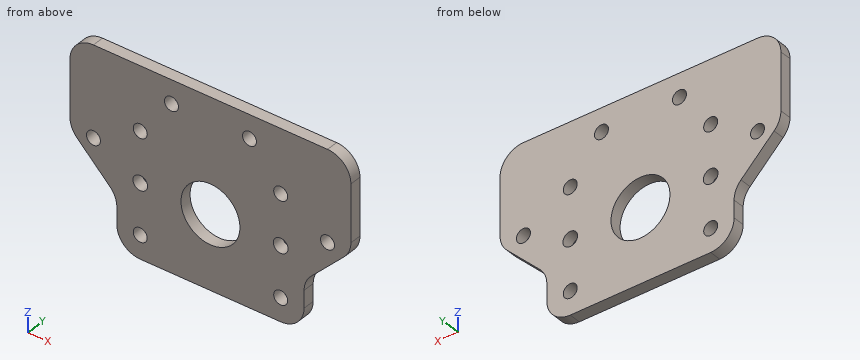
from build123d import *

# Parameters (mm, degrees)
SKETCH1_R           = 8
BOSS_EXTRUDE1_DEPTH = 3.175
SKETCH2_R           = 1.9939
CUT_EXTRUDE1_DEPTH  = 4.175
SKETCH14_R          = 1.89865
M3_TAP_DEPTH        = 4.175
SKETCH15_R          = 1.89865
M5_THROUGH_DEPTH    = 4.175
CUT_EXTRUDE2_DEPTH  = 4.175
FILLET2_R           = 6.35


with BuildPart() as part:
    # Sketch1 → Boss-Extrude1 (new body)
    with BuildSketch(Plane(origin=(0, 0, 0), x_dir=(1, 0, 0), z_dir=(0, 1, 0))):
        Polygon((0, 0), (76.2, 0), (76.2, 50.8), (38.1, 50.8), (0, 50.8), align=None)
        with Locations((38.1, 30.8)):
            Circle(SKETCH1_R, mode=Mode.SUBTRACT)
    extrude(amount=BOSS_EXTRUDE1_DEPTH)

    # Sketch2 → Cut-Extrude1 (cut, through all)
    with BuildSketch(Plane(origin=(0, 3.175, 0), x_dir=(1, 0, 0), z_dir=(0, 1, 0))):
        with Locations((19.05, 30.8)):
            Circle(SKETCH2_R)
        with Locations((57.15, 30.8)):
            Circle(SKETCH2_R)
    extrude(amount=-CUT_EXTRUDE1_DEPTH, mode=Mode.SUBTRACT)

    # Sketch14 → M3-tap (cut, through all)
    with BuildSketch(Plane.XZ):
        with Locations((57.15, -44.45)):
            Circle(SKETCH14_R)
        with Locations((19.05, -44.45)):
            Circle(SKETCH14_R)
        with Locations((19.05, -17.15)):
            Circle(SKETCH14_R)
        with Locations((57.15, -17.15)):
            Circle(SKETCH14_R)
    extrude(amount=-M3_TAP_DEPTH, mode=Mode.SUBTRACT)

    # Sketch15 → M5-through (cut, through all)
    with BuildSketch(Plane.XZ):
        with Locations((69.85, -24.45004)):
            Circle(SKETCH15_R)
        with Locations((48.683333333, -6.35)):
            Circle(SKETCH15_R)
        with Locations((27.516666667, -6.35)):
            Circle(SKETCH15_R)
        with Locations((6.35, -24.45004)):
            Circle(SKETCH15_R)
    extrude(amount=-M5_THROUGH_DEPTH, mode=Mode.SUBTRACT)

    # Sketch12 → Cut-Extrude2 (cut, through all)
    with BuildSketch(Plane(origin=(0, 3.175, 0), x_dir=(1, 0, 0), z_dir=(0, 1, 0))):
        Polygon((0, 50.8), (12.7, 50.8), (12.7, 37.15), (0, 24.45), align=None)
        Polygon((63.5, 50.8), (63.5, 37.15), (76.2, 24.45), (76.2, 50.8), align=None)
    extrude(amount=-CUT_EXTRUDE2_DEPTH, mode=Mode.SUBTRACT)

    # Fillet2
    fillet2_edges = [part.edges().sort_by_distance(p)[0] for p in [
        (0, 1.5875, -24.45),
        (12.7, 1.5875, -50.8),
        (12.7, 1.5875, -37.15),
        (63.5, 1.5875, -50.8),
        (76.2, 1.5875, -24.45),
        (63.5, 1.5875, -37.15),
        (76.2, 1.5875, 0),
        (0, 1.5875, 0),
    ]]
    fillet(fillet2_edges, radius=FILLET2_R)


solid = part.part
For this review, take the finished solid that the model builds, in its own axes (mm). Give positions to 0.01 mm unless a question says otherwise; leave off trailing zeros. Order: outer loops, then holes, each group sorted by start corner. A loop starts at its lowest first (then second) coordinate and runs counter-clockwise, first axis right, second up. Notation, with made-up numbers: M 62,36.5 L 82,36.5 A5 ccw 82,45.5 Z; hole C 48,-24 d9. An arc over 180 degrees is marked long. Answer in a Markdown table with one row per item. Add a question column.
(1) For pin 1 (1 mm diameter, centred on y = 1.5, z = -41, fed in from -X); pin 2 (1 mm diameter, centred on y = 2, z = -42, fed in from +X), all flat-tipped, find the tip position at first contact; note any pin that passes through.
(2) Consider section C-C on z = -17.15. State the section outline as (x, y) points (3 decimals).
(3) Wall thickness on probe 1 along Z at (x, y) = (19.05, 0.85); probe 2 along X at (y, z) = (1.45, -6.5); probe 3 along X at (y, z) = (1.15, -30): over which ranges is each line inside the solid? List them lowest first. Write a range as [from, to].
(4) Consider section A-A on z = -30.8. State the section outline as (x, y) points (3 decimals), and give its area (3 significant figures).
(5) Consider section B-B on x = 33. State the section outline as (y, z) points (3 decimals).
(6) Consider section D-D on y = 2.6. Give the number of separate pieces and of enclosed holes in the cut face, and give its area (3 significant figures).
Evaluation:
| question | item | result |
|---|---|---|
| 1 | pin 1 | stops at x = 12.7 |
| 1 | pin 2 | stops at x = 63.5 |
| 2 | outline | M 0,0 L 17.151,0 L 17.151,3.175 L 0,3.175 Z; M 20.949,0 L 55.251,0 L 55.251,3.175 L 20.949,3.175 Z; M 59.049,0 L 76.2,0 L 76.2,3.175 L 59.049,3.175 Z |
| 3 | probe 1 | z = [-50.8, -46.35], [-42.55, -32.79], [-28.81, -19.05], [-15.25, 0] |
| 3 | probe 2 | x = [0, 25.62], [29.41, 46.79], [50.58, 76.2] |
| 3 | probe 3 | x = [5.55, 17.22], [20.88, 30.14], [46.06, 55.32], [58.98, 70.65] |
| 4 | outline | M 6.35,0 L 17.056,0 L 17.056,3.175 L 6.35,3.175 Z; M 21.044,0 L 30.1,0 L 30.1,3.175 L 21.044,3.175 Z; M 46.1,0 L 55.156,0 L 55.156,3.175 L 46.1,3.175 Z; M 59.144,0 L 69.85,0 L 69.85,3.175 L 59.144,3.175 Z |
| 4 | area | 125 mm^2 |
| 5 | outline | M 0,-50.8 L 3.175,-50.8 L 3.175,-36.964 L 0,-36.964 Z; M 0,-24.636 L 3.175,-24.636 L 3.175,0 L 0,0 Z |
| 6 | separate pieces | 1 |
| 6 | enclosed holes | 11 |
| 6 | area | 3,010 mm^2 |
